```python
from build123d import *

# Parameters (mm, degrees)
SKETCH1_W               = 8
SKETCH1_H               = 8
BOSS_EXTRUDE1_DEPTH     = 3
CUT_EXTRUDE1_DEPTH      = 12.704699911
CUT_EXTRUDE1_DEPTH_BACK = 12.704699911
CUT_EXTRUDE2_DEPTH      = 11
SKETCH4_R               = 1.8
CUT_EXTRUDE3_DEPTH      = 0.8
SKETCH5_W               = 8
SKETCH5_H               = 1
BOSS_EXTRUDE2_DEPTH     = 2
FILLET1_R               = 4
CUT_EXTRUDE4_DEPTH      = 0.4


with BuildPart() as part:
    # Sketch1 → Boss-Extrude1 (new body)
    with BuildSketch(Plane(origin=(0, 0, 0), x_dir=(1, 0, 0), z_dir=(0, 1, 0))):
        with Locations((4, 4)):
            Rectangle(SKETCH1_W, SKETCH1_H)
    extrude(amount=BOSS_EXTRUDE1_DEPTH)

    # Sketch2 → Cut-Extrude1 (cut, two sides: drawn at the far end of the back side and taken through both)
    with BuildSketch(Plane.XY.offset(-CUT_EXTRUDE1_DEPTH_BACK)):
        Polygon((0, 0), (0.6, 3), (0, 3), align=None)
        Polygon((8, 0), (7.4, 3), (8, 3), align=None)
    extrude(amount=CUT_EXTRUDE1_DEPTH + CUT_EXTRUDE1_DEPTH_BACK, mode=Mode.SUBTRACT)

    # Sketch3 → Cut-Extrude2 (cut)
    with BuildSketch(Plane(origin=(0, 0, 0), x_dir=(0, 0, -1), z_dir=(1, 0, 0))):
        Polygon((0, 0), (0.6, 3), (0, 3), align=None)
        Polygon((8, 3), (7.4, 3), (8, 0), align=None)
    extrude(amount=CUT_EXTRUDE2_DEPTH, mode=Mode.SUBTRACT)

    # Sketch4 → Cut-Extrude3 (cut)
    with BuildSketch(Plane.XZ):
        with Locations(Location((4, -3.75, 0), (0, 0, 270))):
            Circle(SKETCH4_R)
    extrude(amount=-CUT_EXTRUDE3_DEPTH, mode=Mode.SUBTRACT)

    # Sketch5 → Boss-Extrude2 (add)
    with BuildSketch(Plane.XZ):
        with Locations((4, -7.5)):
            Rectangle(SKETCH5_W, SKETCH5_H)
    extrude(amount=BOSS_EXTRUDE2_DEPTH)

    # Fillet1
    # the kernel refuses this fillet: 4 mm, written as the material it takes off along each edge
    with BuildSketch(Plane(origin=(8, -2, -16.660254038), x_dir=(0, 1, 0), z_dir=(0, 0, 1)), Plane(origin=(0, -2, 1.660254038), x_dir=(0, 1, 0), z_dir=(0, 0, -1))) as fillet1_piece_1:
        with BuildLine():
            CenterArc((4, 3.464101615), FILLET1_R, 180, 60)
            Line((0, 3.464101615), (-0.08, 3.464101615))
            Line((-0.08, 3.464101615), (-0.08, 0))
            Line((-0.08, 0), (0, -0.08))
            ThreePointArc((0, -0.08), (1, -0.08), (1.96, -0.069282032))
            Line((1.96, -0.069282032), (2, 0))
        make_face()
    extrude(amount=18.320508076, mode=Mode.SUBTRACT)

    # Sketch6 → Cut-Extrude4 (cut)
    with BuildSketch(Plane(origin=(0, 3, 0), x_dir=(1, 0, 0), z_dir=(0, 1, 0))):
        with BuildLine():
            Line((2.312898911, 2.041410717), (2.312898911, 6.041410717))
            Line((2.312898911, 6.041410717), (3.991584808, 6.041410717))
            add(Edge.make_bspline(
                [(3.991584808, 6.041410717), (4.042601732, 6.041096301), (4.140920681, 6.040490364), (4.283109063, 6.036071747), (4.414238667, 6.026814487), (4.534891188, 6.016330564), (4.644487122, 6.001077132), (4.74345979, 5.982803671), (4.831642566, 5.961627249), (4.910322089, 5.936265049), (4.982061831, 5.90723713), (5.04889092, 5.87268574), (5.111544162, 5.83220454), (5.170983849, 5.787188805), (5.227461685, 5.737569368), (5.279429347, 5.682033053), (5.32779225, 5.621406813), (5.372511371, 5.556195062), (5.411906117, 5.48668575), (5.447902572, 5.415111184), (5.477205044, 5.340709703), (5.50140862, 5.263831792), (5.52074281, 5.184644366), (5.534162371, 5.102946099), (5.542540058, 5.018884869), (5.543287935, 4.962103945), (5.543668142, 4.93323764)],
                knots=[0, 0, 0, 0, 1.675828044, 3.229627355, 4.67171229, 5.993455049, 7.206927059, 8.304770529, 9.29850117, 10.183580433, 11.017754134, 11.837875825, 12.650738409, 13.464925643, 14.285328857, 15.117007378, 15.959673368, 16.830859064, 17.711229498, 18.58228265, 19.460420693, 20.334473227, 21.228207035, 22.135446768, 23.052097822, 24, 24, 24, 24], degree=3))
            add(Edge.make_bspline(
                [(5.543668142, 4.93323764), (5.542962916, 4.896874176), (5.541584712, 4.825809944), (5.528901745, 4.721651895), (5.5100643, 4.622136315), (5.483211668, 4.527125334), (5.446289845, 4.437736414), (5.403428122, 4.352717347), (5.352308317, 4.272356517), (5.293277733, 4.19745058), (5.226389218, 4.127933229), (5.151349641, 4.065235076), (5.06869476, 4.009111084), (4.977924564, 3.959884897), (4.879671091, 3.917801842), (4.77350828, 3.882394441), (4.659916733, 3.853576761), (4.580902516, 3.840017181), (4.540463013, 3.833077384)],
                knots=[0, 0, 0, 0, 1.05911256, 2.069797862, 3.05271628, 4.008392045, 4.940519534, 5.866323021, 6.779546087, 7.71056835, 8.640711998, 9.585328432, 10.554502533, 11.547017206, 12.589327225, 13.664782803, 14.804835066, 16, 16, 16, 16], degree=3))
            add(Edge.make_bspline(
                [(4.540463013, 3.833077384), (4.579572554, 3.807174767), (4.656115253, 3.756479818), (4.762017587, 3.672984601), (4.857092756, 3.585349912), (4.929078878, 3.507419696), (4.984392794, 3.438888442), (5.028929947, 3.378950347), (5.076970406, 3.309970293), (5.128042999, 3.231910907), (5.183657562, 3.145462828), (5.241745689, 3.049302835), (5.303522957, 2.944368887), (5.345058377, 2.871067212), (5.366584808, 2.833077384)],
                knots=[0, 0, 0, 0, 1.285445069, 2.515791127, 3.691898215, 4.826622834, 5.420063933, 6.105349801, 6.873086501, 7.723915395, 8.66222816, 9.690593598, 10.803111229, 12, 12, 12, 12], degree=3))
            Line((5.366584808, 2.833077384), (5.851360449, 2.041410717))
            Line((5.851360449, 2.041410717), (4.952321988, 2.041410717))
            Line((4.952321988, 2.041410717), (4.383411731, 2.949263281))
            add(Edge.make_bspline(
                [(4.383411731, 2.949263281), (4.357283981, 2.985622121), (4.307400733, 3.055038622), (4.235391184, 3.153681722), (4.169508837, 3.241491798), (4.111507042, 3.319740728), (4.058450932, 3.386209972), (4.011951502, 3.442057857), (3.972955886, 3.488482798), (3.928832249, 3.534515131), (3.877499082, 3.581823547), (3.813952721, 3.627691749), (3.748696505, 3.664257396), (3.678779681, 3.692157844), (3.597922987, 3.71161189), (3.500720436, 3.724006591), (3.384115753, 3.733151261), (3.299833928, 3.733519777), (3.254405321, 3.73371841)],
                knots=[0, 0, 0, 0, 1.465447777, 2.797841088, 3.997266218, 5.05856206, 5.985598736, 6.780315439, 7.437430484, 7.969193402, 8.866571936, 9.718200644, 10.52825214, 11.309096006, 12.174169268, 13.242355782, 14.513606761, 16, 16, 16, 16], degree=3))
            Line((3.254405321, 3.73371841), (3.08212968, 3.73371841))
            Line((3.08212968, 3.73371841), (3.08212968, 2.041410717))
            Line((3.08212968, 2.041410717), (2.312898911, 2.041410717))
        make_face()
        with BuildLine():
            Line((3.08212968, 4.400385076), (3.701520706, 4.400385076))
            add(Edge.make_bspline(
                [(3.701520706, 4.400385076), (3.749332843, 4.400487541), (3.840423044, 4.400682752), (3.969955122, 4.403510317), (4.085670885, 4.405910235), (4.186877859, 4.411940131), (4.274028855, 4.417916326), (4.346774263, 4.425683211), (4.405726987, 4.434863419), (4.464610849, 4.449136231), (4.52492793, 4.474003789), (4.589214527, 4.509422512), (4.644158691, 4.555370201), (4.691753027, 4.608490376), (4.728060837, 4.670937972), (4.756498441, 4.739930879), (4.770916908, 4.817002181), (4.773239296, 4.87042263), (4.774437372, 4.89798123)],
                knots=[0, 0, 0, 0, 1.697953026, 3.23488743, 4.60134403, 5.807846676, 6.835100678, 7.703488618, 8.405232423, 8.952775585, 9.851109663, 10.713519226, 11.549115941, 12.382556273, 13.233359028, 14.101746968, 15.020727134, 16, 16, 16, 16], degree=3))
            add(Edge.make_bspline(
                [(4.774437372, 4.89798123), (4.773074786, 4.928811222), (4.770445895, 4.98829272), (4.749714088, 5.072935459), (4.713527564, 5.147705664), (4.663829732, 5.212726785), (4.601441933, 5.267631557), (4.527131165, 5.311213996), (4.441449505, 5.343672387), (4.379650359, 5.355659208), (4.347354039, 5.361923538)],
                knots=[0, 0, 0, 0, 1.062977961, 2.050844577, 2.982300261, 3.90936959, 4.856017476, 5.831122378, 6.86654153, 8, 8, 8, 8], degree=3))
            add(Edge.make_bspline(
                [(4.347354039, 5.361923538), (4.336678458, 5.363096555), (4.311375089, 5.365876852), (4.266692338, 5.367662514), (4.20955971, 5.370407271), (4.139285669, 5.371528992), (4.056498042, 5.373495271), (3.960867626, 5.373856329), (3.852698247, 5.375009885), (3.776307493, 5.374835906), (3.735975834, 5.374744051)],
                knots=[0, 0, 0, 0, 0.42127143, 0.998501726, 1.753681744, 2.66564073, 3.755712164, 5.002818897, 6.417592707, 8, 8, 8, 8], degree=3))
            Line((3.735975834, 5.374744051), (3.08212968, 5.374744051))
            Line((3.08212968, 5.374744051), (3.08212968, 4.400385076))
        make_face(mode=Mode.SUBTRACT)
    extrude(amount=-CUT_EXTRUDE4_DEPTH, mode=Mode.SUBTRACT)


solid = part.part
```
Work out the finished part from the listing and answer in its coordinate system (mm). A direction names the side the tool comes from. Give positions to 0.01 mm unless a question says otherwise; leave off trailing zeros. Loops run counter-clockwise (first coordinate to the right, second up) from the corner with the lowest first, then second, coordinate; pieces in that order, holes last. Notation, with made-up numbers: M 44,38.25 L 59,38.25 A9 ccw 59,47.25 Z; hole C -12,36.25 d7. An arc over 180 degrees is marked long. One line per item, written item: value. Start each with the question number.
1. Find section A-A (x = 6.5). Give the vertices of the cut face in (y, z), and give its area (3 significant figures).
2. Find the intervals of material crossed by probe 1 along X at (y, z) = (2.7, -4.5); probe 2 along Y at (x, z) = (5.75, -1.5); probe 3 along X at (y, z) = (0.45, -3.75), in increasing order.
3. Find section B-B (z = -1.75). Give the vertices of the cut face in (x, y).
4. Find section D-D (x = 1.75). Give the vertices of the cut face in (y, z), and give its area (3 significant figures).
5. Each of these flat-tipped pins is pushed along its axis until it touches: P1, Ø4, axis at x = 4.5, z = -4, coming from the -Y side; P2, Ø1, axis at x = 4.5, y = -1.5, coming from the +Z side; P3, Ø4.5, axis at x = 4, z = -3.75, coming from the +Y side; P4, Ø3, axis at x = 5.5, y = 2, coming from the -Z side. Where does it stop, or does it pass through?
6. Determine the mould class of faces 4 (the face through (4, 2.6, -4)), 5 (the face through (3.9, 1.5, -0.3)), 6 (the face through (6.51, -1.48, -7.51)) for opening direction Z: released by +Z, released by -Z, zero draft, split by the parting line, or undercut.
7. Find section C-C (y = -1.2). Give the vertices of the cut face in (x, z).
8. Which of the six approach directions +Z, -Z, +X, -X, +Y, -Y give full straight-line access (tool end or side, diameter ignored) to faces 1 (the face through (4, 3, -5)), 2 (the face through (4, -1, -7)), 3 (the face through (4.541, 0.394, -5.467))?
Reported:
1. outline: M -1.48,-8 L 0,-8 L 3,-7.4 L 3,-0.6 L 0,0 L 0,-7 L -1.48,-7 Z
1. area: 23.7 mm²
2. probe 1: x = 0.54 to 2.31, 3.08 to 4.57, 5.47 to 7.46
2. probe 2: y = 0 to 3
2. probe 3: x = 0.09 to 2.2, 5.8 to 7.91
3. outline: M 0,0 L 8,0 L 7.4,3 L 0.6,3 Z
4. outline: M -1.61,-8 L 0,-8 L 3,-7.4 L 3,-0.6 L 0,0 L 0,-7 L -1.61,-7 Z
4. area: 23.8 mm²
5. P1: stops at y = 0
5. P2: stops at z = -7
5. P3: stops at y = 3
5. P4: stops at z = -7.9
6. face 4: undercut
6. face 5: released by +Z
6. face 6: zero draft
7. outline: M 1.06,-8 L 6.94,-8 L 6.94,-7 L 1.06,-7 Z
8. face 1: +Z, -Z, +X, -X, +Y
8. face 2: +Z, +X, -X, -Y
8. face 3: -Y
